Read the model definition and answer for the solid it produces. Units are mm, in the model's axes. Face numbers are marked on the shaded views. Coordinates: 2 decimals unless noted, no trailing zeros. Write each loop counter-clockwise with the first axis right and the second up, starting at its lowest first coordinate (ties: lowest second). Pieces come first, ordered by that corner, then holes.
1) The part is cut by section D-D (y = 1.5). Determine the outline of the cut face in (x, z), then the cut area to 3 significant figures.
2) The part is cut by section A-A (y = 3.75). Determine the outline of the cut face in (x, z), then the cut area to 3 significant figures.
3) Determine the mould class of the marked faces 1 and 2 for opening direction X: +X half, -X half, draft (parallel to the pull), parting line (faces both ways), or undercut.
4) Each of these flat-tipped pins is pushed along its axis until it touches: pin 1 Ø5 at (x, z) = (-2.5, 11.5) entering from -Y; pin 2 Ø3 at (x, z) = (-2, 11.5) entering from -Y. Where does it stop, or does it pass through?
5) Find the intervals of material crossed by line 1 (Y direction, x = 0, z = 23.5); line 2 (X direction, y = 4, z = 10.5); line 3 (X direction, y = 3, z = 21), in increasing order.
6) The part is cut by section C-C (x = 0). Determine the outline of the cut face in (y, z), then the cut area to 3 significant figures.
from build123d import *

# Parameters (mm, degrees)
F1_DEPTH = 40
F2_R     = 0.79999


# Not quite as in the source:
# - a fillet or chamfer is up to 0.001 mm smaller than in the source, because OpenCascade refuses the exact size


with BuildPart() as f1:
    # F0 (on Top) → F1 (new body)
    with BuildSketch(Plane.XY):
        with BuildLine():
            ThreePointArc((-8.0155554774, -0.7438886939), (0.8184709888, 8.008283539), (7.699350622, -2.35))
            Line((7.699350622, -2.35), (9.3594871654, -2.35))
            ThreePointArc((9.3594871654, -2.35), (0, 9.65), (-9.3594871654, -2.35))
            Line((-9.3594871654, -2.35), (-7.699350622, -2.35))
            Line((-7.699350622, -2.35), (-5.5929206907, -1.4413775962))
            Line((-5.5929206907, -1.4413775962), (-6.2266466845, 0.0277688788))
            Line((-6.2266466845, 0.0277688788), (-8.0155554774, -0.7438886939))
        make_face()
    extrude(amount=F1_DEPTH)

    # F2 (radius 0.8 in the source; OpenCascade refuses exactly that, so slightly less here)
    f2_edges = [f1.edges().sort_by_distance(p)[0] for p in [
        (-7.699351, -2.35, 20),
        (7.699351, -2.35, 20),
        (9.359487, -2.35, 20),
        (-9.359487, -2.35, 20),
    ]]
    fillet(f2_edges, radius=F2_R)


solid = f1.part
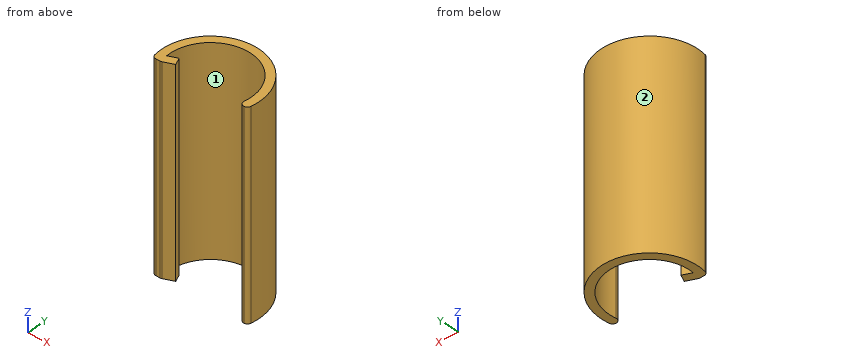
Reported:
1. outline: (-9.53, 0) - (-7.91, 0) - (-7.91, 40) - (-9.53, 40) - close; (7.91, 0) - (9.53, 0) - (9.53, 40) - (7.91, 40) - close
1. area: 130 mm2
2. outline: (-8.89, 0) - (-7.12, 0) - (-7.12, 40) - (-8.89, 40) - close; (7.12, 0) - (8.89, 0) - (8.89, 40) - (7.12, 40) - close
2. area: 141 mm2
3. face 1: undercut
3. face 2: parting line
4. pin 1: stops at y = 6.31
4. pin 2: stops at y = 7.25
5. line 1: y = 8.05 to 9.65
5. line 2: x = -8.78 to -6.99, 6.99 to 8.78
5. line 3: x = -9.17 to -7.47, 7.47 to 9.17
6. outline: (8.05, 0) - (9.65, 0) - (9.65, 40) - (8.05, 40) - close
6. area: 64.0 mm2
